Input: part model. Units: mm. Frame: model coordinates. A direction names the side the tool comes from. Coordinates: 2 decimals unless noted, no trailing zeros. Write each loop counter-clockwise with the first axis right and the second up, starting at its lowest first coordinate (ties: lowest second). Pieces come first, ordered by that corner, then holes. Notation, with made-up numbers: (6.25, 82.25) -> (50.25, 82.25) arc R25 cw to (50.25, 101.25) -> close; hole circle Ø2 at (32, 79). An arc over 180 degrees is marked (long way). Use one line per item in the form item = value. Start each with the question number.
(1) Ray query, line 1 along Z through (x, y) = (-66.53, 4.1); line 2 along Z through (x, y) = (66.53, 2.25); line 3 along X through (y, z) = (5.1, -26.5). Return the intervals inside material, ascending.
(2) Cut plane A-A on x = -34.5. Return the cut outline in (y, z), plus the area to 3 significant figures.
(3) Pull-direction query (X, two-part tool) for faces 1 (the face through (-1, 0, -1)), 2 (the face through (12.35, 1.9, -54.18)), 3 (the face through (12.35, 1.9, 54.18)); classes: released by +X, released by -X, zero draft, split by the parting line, or undercut.
(4) First-contact query: pin 1 (5 mm diameter, centred on x = -66.53, z = 18.83, fed in from +Y); pin 2 (1.6 mm diameter, centred on x = -13.5, y = 2.5, fed in from +Z); pin 3 (3.5 mm diameter, centred on x = -66.53, z = 0, fed in from -Y). Flat tips, straight axial feed; report the tip coordinate or a pass-through.
(5) Set-up query: faces 4 (the face through (-41, 3, 52.3)), 5 (the face through (-68.48, 1.48, -37.23)), 6 (the face through (-41, 3, -52.3)). Return all of +Z, -Z, +X, -X, +Y, -Y with unobstructed straight access to the full face (end or side cutting, diameter ignored); none if empty.
```python
from build123d import *

# Parameters (mm, degrees)
SKETCH_1_W             = 138.06
SKETCH_1_H             = 113
EXTRUDE_301_DEPTH      = 5
EXTRUDE_2092_DEPTH     = 0.7
SKETCH_3_R             = 1.575
CUT_EXTRUDE_2766_DEPTH = 4.2
CUT_EXTRUDE_3301_REACH = 91.386
SKETCH_4_R             = 1.05
SKETCH_5_R             = 2
CUT_EXTRUDE_3811_DEPTH = 3
CHAMFER_3856_SIZE      = 0.5


with BuildPart() as part:
    # Sketch 1 → Extrude 301 (new body)
    with BuildSketch(Plane(origin=(0, 0, 0), x_dir=(1, 0, 0), z_dir=(0, 1, 0))):
        Rectangle(SKETCH_1_W, SKETCH_1_H)
    extrude(amount=EXTRUDE_301_DEPTH)

    # Sketch 2 → Extrude 2092 (add)
    with BuildSketch(Plane(origin=(0, 5, 0), x_dir=(1, 0, 0), z_dir=(0, 1, 0))):
        Polygon((-62.35, -2.575), (-63.35, -2.575), (-63.35, -51.6), (-61.525, -51.6), (-61.525, -50.6), (-62.35, -50.6), align=None)
        Polygon((-61.525, 45.45), (-61.525, 46.45), (-63.35, 46.45), (-63.35, -2.575), (-62.35, -2.575), (-62.35, 45.45), align=None)
        Polygon((-59.7, -2.575), (-59.7, 46.45), (-61.525, 46.45), (-61.525, 45.45), (-60.7, 45.45), (-60.7, -2.575), align=None)
        Polygon((-59.7, -51.6), (-59.7, -2.575), (-60.7, -2.575), (-60.7, -50.6), (-61.525, -50.6), (-61.525, -51.6), align=None)
        Polygon((62.35, 45.45), (62.35, -2.575), (63.35, -2.575), (63.35, 46.45), (61.525, 46.45), (61.525, 45.45), align=None)
        Polygon((59.7, -2.575), (60.7, -2.575), (60.7, 45.45), (61.525, 45.45), (61.525, 46.45), (59.7, 46.45), align=None)
        Polygon((61.525, -51.6), (61.525, -50.6), (60.7, -50.6), (60.7, -2.575), (59.7, -2.575), (59.7, -51.6), align=None)
        Polygon((62.35, -50.6), (61.525, -50.6), (61.525, -51.6), (63.35, -51.6), (63.35, -2.575), (62.35, -2.575), align=None)
    extrude(amount=EXTRUDE_2092_DEPTH)

    # Fillet 2147: read off the stored shape, not the designer's step
    # Fillet 2147: loft between two sections, ruled curve by curve
    fillet_2147_from = [
        Edge.make_line((-62.35, 5.2, -45.45), (-60.7, 5.2, -45.45)),
        Edge.make_line((-60.7, 5.2, -45.45), (-60.7, 5.2, 50.6)),
        Edge.make_line((-60.7, 5.2, 50.6), (-62.35, 5.2, 50.6)),
        Edge.make_line((-62.35, 5.2, -45.45), (-62.35, 5.2, 50.6)),
    ]
    fillet_2147_to = [
        Edge.make_line((-62.85, 5.7, -45.95), (-60.2, 5.7, -45.95)),
        Edge.make_line((-60.2, 5.7, -45.95), (-60.2, 5.7, 51.1)),
        Edge.make_line((-60.2, 5.7, 51.1), (-62.85, 5.7, 51.1)),
        Edge.make_line((-62.85, 5.7, -45.95), (-62.85, 5.7, 51.1)),
    ]
    fillet_2147 = Solid(Shell([*[Face.make_surface_from_curves(fillet_2147_from[k], fillet_2147_to[k]) for k in range(4)], Face(Wire(fillet_2147_from)), Face(Wire(fillet_2147_to))]))
    add(fillet_2147, mode=Mode.SUBTRACT)

    # Fillet 2335: read off the stored shape, not the designer's step
    # Fillet 2335: loft between two sections, ruled curve by curve
    fillet_2335_from = [
        Edge.make_line((60.7, 5.2, -45.45), (62.35, 5.2, -45.45)),
        Edge.make_line((62.35, 5.2, -45.45), (62.35, 5.2, 50.6)),
        Edge.make_line((62.35, 5.2, 50.6), (60.7, 5.2, 50.6)),
        Edge.make_line((60.7, 5.2, -45.45), (60.7, 5.2, 50.6)),
    ]
    fillet_2335_to = [
        Edge.make_line((60.2, 5.7, -45.95), (62.85, 5.7, -45.95)),
        Edge.make_line((62.85, 5.7, -45.95), (62.85, 5.7, 51.1)),
        Edge.make_line((62.85, 5.7, 51.1), (60.2, 5.7, 51.1)),
        Edge.make_line((60.2, 5.7, -45.95), (60.2, 5.7, 51.1)),
    ]
    fillet_2335 = Solid(Shell([*[Face.make_surface_from_curves(fillet_2335_from[k], fillet_2335_to[k]) for k in range(4)], Face(Wire(fillet_2335_from)), Face(Wire(fillet_2335_to))]))
    add(fillet_2335, mode=Mode.SUBTRACT)

    # Sketch 3 → Cut-Extrude 2766 (cut)
    with BuildSketch(Plane(origin=(0, 0, -56.5), x_dir=(-1, 0, 0), z_dir=(0, 0, -1))):
        with Locations((-41.418, 2.5)):
            Circle(SKETCH_3_R)
        with Locations((-13.806, 2.5)):
            Circle(SKETCH_3_R)
        with Locations((13.806, 2.5)):
            Circle(SKETCH_3_R)
        with Locations((41.418, 2.5)):
            Circle(SKETCH_3_R)
    cut_extrude_2766 = extrude(amount=-CUT_EXTRUDE_2766_DEPTH, mode=Mode.SUBTRACT)

    # Mirror 1: Cut-Extrude 2766 across plane
    add(cut_extrude_2766.mirror(Plane(origin=(0, 0, 0), x_dir=(1, 0, 0), z_dir=(0, 0, -1))), mode=Mode.SUBTRACT)

    # Sketch 4 → Cut-Extrude 3301 (cut, up to next)
    with BuildSketch(Plane.XZ, mode=Mode.PRIVATE) as cut_extrude_3301_sk1:
        with Locations(Location((-66.53, 37.666666667, 0), (0, 0, 270))):
            Circle(SKETCH_4_R)
    cut_extrude_3301_tool1 = extrude(cut_extrude_3301_sk1.sketch, amount=-CUT_EXTRUDE_3301_REACH, mode=Mode.PRIVATE) & part.part
    # Sketch 4 → Cut-Extrude 3301 (cut, up to next)
    with BuildSketch(Plane.XZ, mode=Mode.PRIVATE) as cut_extrude_3301_sk2:
        with Locations(Location((-66.53, 18.833333333, 0), (0, 0, 270))):
            Circle(SKETCH_4_R)
    cut_extrude_3301_tool2 = extrude(cut_extrude_3301_sk2.sketch, amount=-CUT_EXTRUDE_3301_REACH, mode=Mode.PRIVATE) & part.part
    # Sketch 4 → Cut-Extrude 3301 (cut, up to next)
    with BuildSketch(Plane.XZ, mode=Mode.PRIVATE) as cut_extrude_3301_sk3:
        with Locations(Location((-66.53, 0, 0), (0, 0, 270))):
            Circle(SKETCH_4_R)
    cut_extrude_3301_tool3 = extrude(cut_extrude_3301_sk3.sketch, amount=-CUT_EXTRUDE_3301_REACH, mode=Mode.PRIVATE) & part.part
    # Sketch 4 → Cut-Extrude 3301 (cut, up to next)
    with BuildSketch(Plane.XZ, mode=Mode.PRIVATE) as cut_extrude_3301_sk4:
        with Locations(Location((-66.53, -18.833333333, 0), (0, 0, 270))):
            Circle(SKETCH_4_R)
    cut_extrude_3301_tool4 = extrude(cut_extrude_3301_sk4.sketch, amount=-CUT_EXTRUDE_3301_REACH, mode=Mode.PRIVATE) & part.part
    # Sketch 4 → Cut-Extrude 3301 (cut, up to next)
    with BuildSketch(Plane.XZ, mode=Mode.PRIVATE) as cut_extrude_3301_sk5:
        with Locations(Location((-66.53, -37.666666667, 0), (0, 0, 270))):
            Circle(SKETCH_4_R)
    cut_extrude_3301_tool5 = extrude(cut_extrude_3301_sk5.sketch, amount=-CUT_EXTRUDE_3301_REACH, mode=Mode.PRIVATE) & part.part
    # Sketch 4 → Cut-Extrude 3301 (cut, up to next)
    with BuildSketch(Plane.XZ, mode=Mode.PRIVATE) as cut_extrude_3301_sk6:
        with Locations(Location((66.53, -37.666666667, 0), (0, 0, 270))):
            Circle(SKETCH_4_R)
    cut_extrude_3301_tool6 = extrude(cut_extrude_3301_sk6.sketch, amount=-CUT_EXTRUDE_3301_REACH, mode=Mode.PRIVATE) & part.part
    # Sketch 4 → Cut-Extrude 3301 (cut, up to next)
    with BuildSketch(Plane.XZ, mode=Mode.PRIVATE) as cut_extrude_3301_sk7:
        with Locations(Location((66.53, -18.833333333, 0), (0, 0, 270))):
            Circle(SKETCH_4_R)
    cut_extrude_3301_tool7 = extrude(cut_extrude_3301_sk7.sketch, amount=-CUT_EXTRUDE_3301_REACH, mode=Mode.PRIVATE) & part.part
    # Sketch 4 → Cut-Extrude 3301 (cut, up to next)
    with BuildSketch(Plane.XZ, mode=Mode.PRIVATE) as cut_extrude_3301_sk8:
        with Locations(Location((66.53, 0, 0), (0, 0, 270))):
            Circle(SKETCH_4_R)
    cut_extrude_3301_tool8 = extrude(cut_extrude_3301_sk8.sketch, amount=-CUT_EXTRUDE_3301_REACH, mode=Mode.PRIVATE) & part.part
    # Sketch 4 → Cut-Extrude 3301 (cut, up to next)
    with BuildSketch(Plane.XZ, mode=Mode.PRIVATE) as cut_extrude_3301_sk9:
        with Locations(Location((66.53, 18.833333333, 0), (0, 0, 270))):
            Circle(SKETCH_4_R)
    cut_extrude_3301_tool9 = extrude(cut_extrude_3301_sk9.sketch, amount=-CUT_EXTRUDE_3301_REACH, mode=Mode.PRIVATE) & part.part
    # Sketch 4 → Cut-Extrude 3301 (cut, up to next)
    with BuildSketch(Plane.XZ, mode=Mode.PRIVATE) as cut_extrude_3301_sk10:
        with Locations(Location((66.53, 37.666666667, 0), (0, 0, 270))):
            Circle(SKETCH_4_R)
    cut_extrude_3301_tool10 = extrude(cut_extrude_3301_sk10.sketch, amount=-CUT_EXTRUDE_3301_REACH, mode=Mode.PRIVATE) & part.part
    add(cut_extrude_3301_tool1.solids().sort_by_distance((-66.53, 0, 37.666667))[0], mode=Mode.SUBTRACT)
    add(cut_extrude_3301_tool2.solids().sort_by_distance((-66.53, 0, 18.833333))[0], mode=Mode.SUBTRACT)
    add(cut_extrude_3301_tool3.solids().sort_by_distance((-66.53, 0, 0))[0], mode=Mode.SUBTRACT)
    add(cut_extrude_3301_tool4.solids().sort_by_distance((-66.53, 0, -18.833333))[0], mode=Mode.SUBTRACT)
    add(cut_extrude_3301_tool5.solids().sort_by_distance((-66.53, 0, -37.666667))[0], mode=Mode.SUBTRACT)
    add(cut_extrude_3301_tool6.solids().sort_by_distance((66.53, 0, -37.666667))[0], mode=Mode.SUBTRACT)
    add(cut_extrude_3301_tool7.solids().sort_by_distance((66.53, 0, -18.833333))[0], mode=Mode.SUBTRACT)
    add(cut_extrude_3301_tool8.solids().sort_by_distance((66.53, 0, 0))[0], mode=Mode.SUBTRACT)
    add(cut_extrude_3301_tool9.solids().sort_by_distance((66.53, 0, 18.833333))[0], mode=Mode.SUBTRACT)
    add(cut_extrude_3301_tool10.solids().sort_by_distance((66.53, 0, 37.666667))[0], mode=Mode.SUBTRACT)

    # Sketch 5 → Cut-Extrude 3811 (cut)
    with BuildSketch(Plane.XZ):
        with Locations(Location((-66.53, 37.666666667, 0), (0, 0, 270))):
            Circle(SKETCH_5_R)
        with Locations(Location((-66.53, 18.833333333, 0), (0, 0, 270))):
            Circle(SKETCH_5_R)
        with Locations(Location((-66.53, 0, 0), (0, 0, 270))):
            Circle(SKETCH_5_R)
        with Locations(Location((-66.53, -18.833333333, 0), (0, 0, 270))):
            Circle(SKETCH_5_R)
        with Locations(Location((-66.53, -37.666666667, 0), (0, 0, 270))):
            Circle(SKETCH_5_R)
        with Locations(Location((66.53, -37.666666667, 0), (0, 0, 90))):
            Circle(SKETCH_5_R)
        with Locations(Location((66.53, -18.833333333, 0), (0, 0, 90))):
            Circle(SKETCH_5_R)
        with Locations(Location((66.53, 0, 0), (0, 0, 90))):
            Circle(SKETCH_5_R)
        with Locations(Location((66.53, 18.833333333, 0), (0, 0, 90))):
            Circle(SKETCH_5_R)
        with Locations(Location((66.53, 37.666666667, 0), (0, 0, 90))):
            Circle(SKETCH_5_R)
    extrude(amount=-CUT_EXTRUDE_3811_DEPTH, mode=Mode.SUBTRACT)

    # Chamfer 3856
    chamfer_3856_edges = [part.edges().sort_by_distance(p)[0] for p in [
        (15.381, 2.5, -56.5),
        (-12.231, 2.5, -56.5),
        (-39.843, 2.5, -56.5),
        (42.993, 2.5, 56.5),
        (15.381, 2.5, 56.5),
        (-12.231, 2.5, 56.5),
        (-39.843, 2.5, 56.5),
        (42.993, 2.5, -56.5),
    ]]
    chamfer(chamfer_3856_edges, length=CHAMFER_3856_SIZE)


solid = part.part
```
Values:
q1.line_1 = -56.5 to -38.72, -36.62 to -19.88, -17.78 to -1.05, 1.05 to 17.78, 19.88 to 36.62, 38.72 to 56.5
q1.line_2 = -56.5 to -39.67, -35.67 to -20.83, -16.83 to -2, 2 to 16.83, 20.83 to 35.67, 39.67 to 56.5
q1.line_3 = -63.35 to -62.35, -60.7 to -59.7, 59.7 to 60.7, 62.35 to 63.35
q2.outline = (0, -56.5) -> (5, -56.5) -> (5, 56.5) -> (0, 56.5) -> close
q2.area = 565 mm2
q3.face_1 = zero draft
q3.face_2 = undercut
q3.face_3 = undercut
q4.pin_1 = 5
q4.pin_2 = 52.3
q4.pin_3 = 3
q5.face_4 = +Z
q5.face_5 = -Y
q5.face_6 = -Z
